from build123d import *

# Parameters (mm, degrees)
F0_R     = 2.5
F1_DEPTH = 1


with BuildPart() as f1:
    # F0 (on Front) → F1 (new body)
    with BuildSketch(Plane.XZ):
        with BuildLine():
            ThreePointArc((12.5, 0), (0, 12.5), (-12.5, 0))
            Line((-12.5, 0), (-12.5, -20))
            ThreePointArc((-12.5, -20), (-10, -22.5), (-7.5, -20))
            ThreePointArc((-7.5, -20), (-5, -17.5), (-2.5, -20))
            ThreePointArc((-2.5, -20), (-1.767767, -21.767767), (0, -22.5))
            ThreePointArc((0, -22.5), (1.767767, -21.767767), (2.5, -20))
            ThreePointArc((2.5, -20), (5, -17.5), (7.5, -20))
            ThreePointArc((7.5, -20), (10, -22.5), (12.5, -20))
            Line((12.5, -20), (12.5, 0))
        make_face()
        with Locations((-5, 0)):
            Circle(F0_R, mode=Mode.SUBTRACT)
        with Locations((5, 0)):
            Circle(F0_R, mode=Mode.SUBTRACT)
    extrude(amount=F1_DEPTH)


solid = f1.part
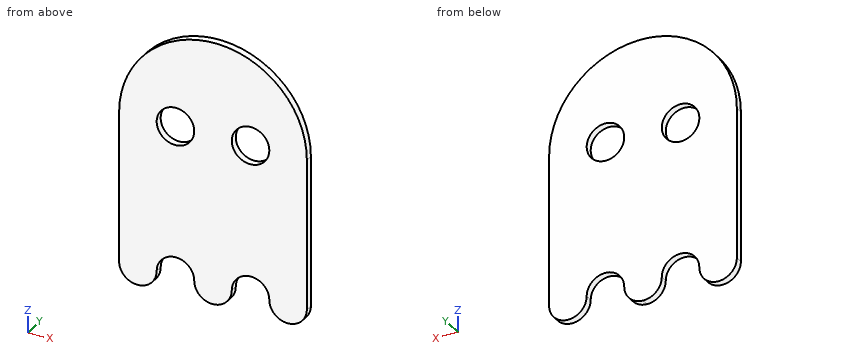
Geometry check sheet. Reference: the model listing, model coordinates, mm. Round coordinates to 2 decimals unless told otherwise and drop trailing zeros. Write each loop counter-clockwise with the first axis right and the second up, starting at its lowest first coordinate (ties: lowest second). Pieces come first, ordered by that corner, then holes.
Item 1: Section check C-C (x = 10). Record the boundary of the cut face in (y, z), plus the area to 3 significant figures.
Determined:
outline: (-1, -22.5) - (0, -22.5) - (0, 7.5) - (-1, 7.5) - close
area: 30.0 mm2
Item 2: Material ranges on line 1 along X through (y, z) = (-0.55, -20); line 2 along X through (y, z) = (-0.7, -1); line 3 along Z through (x, y) = (6.75, -0.3), recorded low to high.
Determined:
line 1: x = -12.5 to -7.5, -2.5 to 2.5, 7.5 to 12.5
line 2: x = -12.5 to -7.29, -2.71 to 2.71, 7.29 to 12.5
line 3: z = -18.21 to -1.79, 1.79 to 10.52
Item 3: Section check D-D (x = 7). Record the boundary of the cut face in (y, z), plus the area to 3 significant figures.
Determined:
outline: (-1, -18.5) - (0, -18.5) - (0, -1.5) - (-1, -1.5) - close; (-1, 1.5) - (0, 1.5) - (0, 10.36) - (-1, 10.36) - close
area: 25.9 mm2
Item 4: Section check A-A (y = -0.7). Record the boundary of the cut face in (x, z).
Determined:
outline: (-12.5, -20) arc R2.5 ccw to (-7.5, -20) arc R2.5 cw to (-2.5, -20) arc R2.5 ccw to (2.5, -20) arc R2.5 cw to (7.5, -20) arc R2.5 ccw to (12.5, -20) - (12.5, 0) arc R12.5 ccw to (-12.5, 0) - close; hole circle Ø5 at (-5, 0); hole circle Ø5 at (5, 0)
Item 5: Section check B-B (x = -5). Record the boundary of the cut face in (y, z).
Determined:
outline: (-1, -17.5) - (0, -17.5) - (0, -2.5) - (-1, -2.5) - close; (-1, 2.5) - (0, 2.5) - (0, 11.46) - (-1, 11.46) - close
